For this review, take the finished solid that the model builds, in its own axes (mm). Face numbers are marked on the shaded views. Coordinates: 2 decimals unless noted, no trailing zeros. Write each loop counter-clockwise with the first axis right and the second up, starting at its lowest first coordinate (ties: lowest second). Pieces come first, ordered by that corner, then holes.
1) Mouldability with a two-part tool opening along X and no side actions: class the marked faces 1 and 2 as pulls with the +X half, pulls with the -X half, needs draft (parallel to the pull), parting line crosses it, or undercut.
2) Insertion check: P1, Ø2, axis at x = 50, z = -28.5, coming from the -Y side; P2, Ø4.5, axis at x = -50, z = 28.5, coming from the +Y side; P3, Ø19.5, axis at x = -7.5, z = -8, coming from the +Y side. Each pin has a flat end and moves straight along its axis. Give the tip position at first contact, or say it passes through.
3) We need section D-D on x = -23.5. Write out the cut boundary in (y, z).
4) We need section A-A on x = -50. Write out the cut boundary in (y, z), then the cut area to 3 significant figures.
5) To check wall thickness, follow line 1 along Z through (x, y) = (-50, 13.2); line 2 along X through (y, z) = (10.4, 28.5); line 3 along Z through (x, y) = (50, 9.4). State the ranges of each line that lie inside material, in increasing order.
6) We need section B-B on z = -28.5. Write out the cut boundary in (x, y).
7) We need section C-C on z = -10.5. Write out the cut boundary in (x, y), then the cut area to 3 significant figures.
from build123d import *

# Parameters (mm, degrees)
SKETCH_W        = 120
SKETCH_H        = 65
PAD007_DEPTH    = 6
POCKET_DEPTH    = 65.001
CHAMFER009_SIZE = 2
SKETCH055_R     = 1.75
POCKET040_DEPTH = 6.001
SKETCH059_R     = 2.8
POCKET041_DEPTH = 2


with BuildPart() as part:
    # Sketch → Pad007 (new body)
    with BuildSketch(Plane.XZ):
        Rectangle(SKETCH_W, SKETCH_H)
    extrude(amount=PAD007_DEPTH)

    # Sketch054 (on Face1 of Pad007) → Pocket (cut, through all)
    with BuildSketch(Plane(origin=(0, 0, 32.5), x_dir=(-1, 0, 0), z_dir=(0, 0, 1))):
        Polygon((-73.60865, -3.669498), (-50.80994, -15.077229), (-50.577229, -15.077229), (-32.5, 3), (32.5, 3), (50.577229, -15.077229), (50.80994, -15.077229), (73.60865, -3.669498), (73.60865, -24.458851), (-87.275108, -33.737259), align=None)
    extrude(amount=-POCKET_DEPTH, mode=Mode.SUBTRACT)

    # Chamfer009
    chamfer009_edges = [part.edges().sort_by_distance(p)[0] for p in [
        (60, -3, -32.5),
        (60, -3, 32.5),
        (60, 0, 0),
        (-60, -3, -32.5),
        (-60, 0, 0),
        (-60, -3, 32.5),
    ]]
    chamfer(chamfer009_edges, length=CHAMFER009_SIZE)

    # Sketch055 → Pocket040 (cut, through all)
    with BuildSketch(Plane(origin=(0, 0, 0), x_dir=(1, 0, 0), z_dir=(0, 1, 0))):
        with Locations((-50, 28.5)):
            Circle(SKETCH055_R)
        with Locations((-50, -28.5)):
            Circle(SKETCH055_R)
        with Locations((50, 28.5)):
            Circle(SKETCH055_R)
        with Locations((50, -28.5)):
            Circle(SKETCH055_R)
    extrude(amount=-POCKET040_DEPTH, mode=Mode.SUBTRACT)

    # Sketch059 (on Face2 of Pocket040) → Pocket041 (cut)
    with BuildSketch(Plane(origin=(0, 0, 0), x_dir=(1, 0, 0), z_dir=(0, 1, 0))):
        with Locations((-50, 28.5)):
            Circle(SKETCH059_R)
        with Locations((-50, -28.5)):
            Circle(SKETCH059_R)
        with Locations((50, 28.5)):
            Circle(SKETCH059_R)
        with Locations((50, -28.5)):
            Circle(SKETCH059_R)
    extrude(amount=-POCKET041_DEPTH, mode=Mode.SUBTRACT)


with BuildPart() as part_1:
    # Body003 placement: moved
    add(part.part.moved(Location((0, 14.15, 0))))


solid = part_1.part
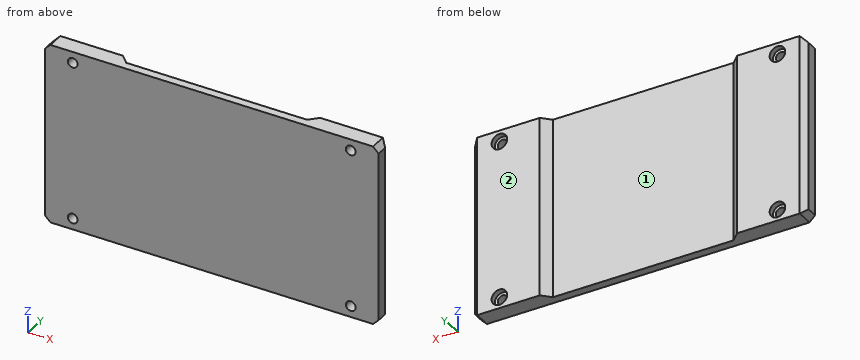
Result:
1. face 1: undercut
1. face 2: needs draft
2. P1: passes through
2. P2: stops at y = 12.15
2. P3: stops at y = 11.15
3. outline: (8.15, -32.5) - (11.15, -32.5) - (11.15, 32.5) - (8.15, 32.5) - close
4. outline: (8.15, -32.5) - (14.15, -32.5) - (14.15, -31.3) - (12.15, -31.3) - (12.15, -30.25) - (8.15, -30.25) - close; (8.15, -26.75) - (12.15, -26.75) - (12.15, -25.7) - (14.15, -25.7) - (14.15, 25.7) - (12.15, 25.7) - (12.15, 26.75) - (8.15, 26.75) - close; (8.15, 30.25) - (12.15, 30.25) - (12.15, 31.3) - (14.15, 31.3) - (14.15, 32.5) - (8.15, 32.5) - close
4. area: 340 mm2
5. line 1: z = -32.5 to -31.3, -25.7 to 25.7, 31.3 to 32.5
5. line 2: x = -60 to -51.75, -48.25 to 48.25, 51.75 to 60
5. line 3: z = -32.5 to -30.25, -26.75 to 26.75, 30.25 to 32.5
6. outline: (-60, 8.15) - (-51.75, 8.15) - (-51.75, 12.15) - (-52.8, 12.15) - (-52.8, 14.15) - (-58, 14.15) - (-60, 12.15) - close; (-48.25, 8.15) - (48.25, 8.15) - (48.25, 12.15) - (47.2, 12.15) - (47.2, 14.15) - (35.5, 14.15) - (32.5, 11.15) - (-32.5, 11.15) - (-35.5, 14.15) - (-47.2, 14.15) - (-47.2, 12.15) - (-48.25, 12.15) - close; (51.75, 8.15) - (60, 8.15) - (60, 12.15) - (58, 14.15) - (52.8, 14.15) - (52.8, 12.15) - (51.75, 12.15) - close
7. outline: (-60, 8.15) - (60, 8.15) - (60, 12.15) - (58, 14.15) - (35.5, 14.15) - (32.5, 11.15) - (-32.5, 11.15) - (-35.5, 14.15) - (-58, 14.15) - (-60, 12.15) - close
7. area: 512 mm2
